```python
from build123d import *

# Parameters (mm, degrees)
F0_R     = 3
F1_DEPTH = 20
F3_DEPTH = 10
F4_R     = 10
F5_DEPTH = 20


with BuildPart() as f1:
    # F0 (on Top) → F1 (new body)
    with BuildSketch(Plane.XY):
        with BuildLine():
            Line((-16.244364, 25.206749), (-21.244364, 25.206749))
            ThreePointArc((-21.244364, 25.206749), (-24.779898, 23.742283), (-26.244364, 20.206749))
            Line((-26.244364, 20.206749), (-26.244364, 15.206749))
            ThreePointArc((-26.244364, 15.206749), (-24.779898, 11.671215), (-21.244364, 10.206749))
            ThreePointArc((-21.244364, 10.206749), (-17.70883, 8.742283), (-16.244364, 5.206749))
            Line((-16.244364, 5.206749), (-16.244364, -4.793251))
            ThreePointArc((-16.244364, -4.793251), (-17.70883, -8.328785), (-21.244364, -9.793251))
            ThreePointArc((-21.244364, -9.793251), (-24.779898, -11.257717), (-26.244364, -14.793251))
            Line((-26.244364, -14.793251), (-26.244364, -19.793251))
            ThreePointArc((-26.244364, -19.793251), (-24.779898, -23.328785), (-21.244364, -24.793251))
            Line((-21.244364, -24.793251), (-16.244364, -24.793251))
            ThreePointArc((-16.244364, -24.793251), (-12.70883, -23.328785), (-11.244364, -19.793251))
            Line((-11.244364, -19.793251), (-11.244364, -17.793251))
            Line((-11.244364, -17.793251), (28.755636, -17.793251))
            Line((28.755636, -17.793251), (28.755636, -19.793251))
            ThreePointArc((28.755636, -19.793251), (30.220102, -23.328785), (33.755636, -24.793251))
            Line((33.755636, -24.793251), (38.755636, -24.793251))
            ThreePointArc((38.755636, -24.793251), (42.29117, -23.328785), (43.755636, -19.793251))
            Line((43.755636, -19.793251), (43.755636, -14.793251))
            ThreePointArc((43.755636, -14.793251), (42.29117, -11.257717), (38.755636, -9.793251))
            ThreePointArc((38.755636, -9.793251), (35.220102, -8.328785), (33.755636, -4.793251))
            Line((33.755636, -4.793251), (33.755636, 5.206749))
            ThreePointArc((33.755636, 5.206749), (35.220102, 8.742283), (38.755636, 10.206749))
            ThreePointArc((38.755636, 10.206749), (42.29117, 11.671215), (43.755636, 15.206749))
            Line((43.755636, 15.206749), (43.755636, 20.206749))
            ThreePointArc((43.755636, 20.206749), (42.29117, 23.742283), (38.755636, 25.206749))
            Line((38.755636, 25.206749), (33.778906, 25.229911))
            ThreePointArc((33.778906, 25.229911), (30.228339, 23.773717), (28.755636, 20.229966))
            Line((28.755636, 20.229966), (28.755636, 18.206749))
            Line((28.755636, 18.206749), (-11.244364, 18.206749))
            Line((-11.244364, 18.206749), (-11.244364, 20.206749))
            ThreePointArc((-11.244364, 20.206749), (-12.70883, 23.742283), (-16.244364, 25.206749))
        make_face()
        with Locations((-19.244364, -17.793251)):
            Circle(F0_R, mode=Mode.SUBTRACT)
        with Locations((36.755636, -17.793251)):
            Circle(F0_R, mode=Mode.SUBTRACT)
        with Locations((-19.244364, 18.206749)):
            Circle(F0_R, mode=Mode.SUBTRACT)
        with Locations((36.755636, 18.206749)):
            Circle(F0_R, mode=Mode.SUBTRACT)
    extrude(amount=F1_DEPTH)

    # F2 (on face) → F3 (cut)
    with BuildSketch(Plane.XY.offset(20)):
        with BuildLine():
            Line((23.755636, 16.206749), (-6.244364, 16.206749))
            ThreePointArc((-6.244364, 16.206749), (-9.779898, 14.742283), (-11.244364, 11.206749))
            Line((-11.244364, 11.206749), (-11.244364, -10.793251))
            ThreePointArc((-11.244364, -10.793251), (-9.779898, -14.328785), (-6.244364, -15.793251))
            Line((-6.244364, -15.793251), (23.755636, -15.793251))
            ThreePointArc((23.755636, -15.793251), (27.29117, -14.328785), (28.755636, -10.793251))
            Line((28.755636, -10.793251), (28.755636, 11.206749))
            ThreePointArc((28.755636, 11.206749), (27.29117, 14.742283), (23.755636, 16.206749))
        make_face()
    extrude(amount=-F3_DEPTH, mode=Mode.SUBTRACT)

    # F4 (on face) → F5 (cut)
    with BuildSketch(Plane.XY.offset(10)):
        with Locations((8.755636, 0.206749)):
            Circle(F4_R)
    extrude(amount=-F5_DEPTH, mode=Mode.SUBTRACT)


solid = f1.part
```
The listing builds one solid part. Answer for the finished solid, in the listing's coordinates (mm). A direction names the side the tool comes from. Give positions to 0.01 mm unless a question says otherwise; leave off trailing zeros. Order: outer loops, then holes, each group sorted by start corner. A loop starts at its lowest first (then second) coordinate and runs counter-clockwise, first axis right, second up.
Item 1: Given pin 1 Ø6 at (x, y) = (11.5, 10) entering from +Z; pin 2 Ø11 at (y, z) = (1, 17) entering from +X; pin 3 Ø6 at (x, z) = (2.5, 9) entering from -Y, each flat-ended and moving along its own axis, determine where each tip first touches the part or whether it passes through.
From the geometry:
pin 1: stops at z = 10
pin 2: stops at x = 33.93
pin 3: stops at y = -17.79
Item 2: The part is cut by section D-D, the plane x = -2. Give the vertices of the cut face in (y, z), and give its area (3 significant figures).
From the geometry:
outline: (-17.79, 0) - (18.21, 0) - (18.21, 20) - (16.21, 20) - (16.21, 10) - (-15.79, 10) - (-15.79, 20) - (-17.79, 20) - close
area: 400 mm2
Item 3: The part is cut by section C-C, the plane z = 11.25. Count the separate pieces of the cut face and the enclosed holes in it, and give its area (3 significant figures).
From the geometry:
separate pieces: 1
enclosed holes: 5
area: 1,130 mm2
Item 4: The part is cut by section B-B, the plane x = 6.5. Give the vertices of the cut face in (y, z), and give its area (3 significant figures).
From the geometry:
outline: (-17.79, 0) - (-9.54, 0) - (-9.54, 10) - (-15.79, 10) - (-15.79, 20) - (-17.79, 20) - close; (9.95, 0) - (18.21, 0) - (18.21, 20) - (16.21, 20) - (16.21, 10) - (9.95, 10) - close
area: 205 mm2
Item 5: For a pull along Y with two mould halves and no side action, classify faces 1 (the face through (9, 16.207, 15)), 2 (the face through (-19, 25.207, 10)), 3 (the face through (8, -17.793, 10)), 4 (the face through (-11.244, -19, 10)) as pulls with the +Y half, pulls with the -Y half, needs draft (parallel to the pull), parting line crosses it, or undercut.
From the geometry:
face 1: undercut
face 2: pulls with the +Y half
face 3: pulls with the -Y half
face 4: needs draft
Item 6: Which of the six approach directions +Z, -Z, +X, -X, +Y, -Y give full straight-line access (tool end or side, diameter ignored) to faces 5 (the face through (-16.244, 0, 10)), 6 (the face through (33.756, 0, 10)), 7 (the face through (9, -15.793, 15)), 8 (the face through (-11.244, 19, 10))?
From the geometry:
face 5: +Z, -Z, -X
face 6: +Z, -Z, +X
face 7: +Z
face 8: +Z, -Z, +Y
Item 7: The part is cut by section A-A, the plane y = -3.5. Give the vertices of the cut face in (x, z), and give its area (3 significant figures).
From the geometry:
outline: (-16.24, 0) - (-0.53, 0) - (-0.53, 10) - (-11.24, 10) - (-11.24, 20) - (-16.24, 20) - close; (18.04, 0) - (33.76, 0) - (33.76, 20) - (28.76, 20) - (28.76, 10) - (18.04, 10) - close
area: 414 mm2
Item 8: Find the intervals of material crossed by probe 1 along Y at (x, z) = (14.5, 13.5); probe 2 along X at (y, z) = (19, 10); probe 3 along X at (y, z) = (3.5, 14.5), in increasing order.
From the geometry:
probe 1: y = -17.79 to -15.79, 16.21 to 18.21
probe 2: x = -26.24 to -22.14, -16.35 to -11.24, 28.76 to 33.86, 39.65 to 43.76
probe 3: x = -16.24 to -11.24, 28.76 to 33.76
